```python
from build123d import *

# Parameters (mm, degrees)
SKETCH2_R          = 11.18
SKETCH2_R_2        = 7.615
CUT_EXTRUDE1_DEPTH = 18
FILLET1_R          = 0.8


with BuildPart() as part:
    # Sketch1 → Revolve1 (revolve)
    with BuildSketch(Plane(origin=(0, 0, 0), x_dir=(0, 0, -1), z_dir=(1, 0, 0)), mode=Mode.PRIVATE) as revolve1_sk:
        with BuildLine():
            Line((12.33, 64), (12.33, 44))
            Line((12.33, 44), (10, 44))
            ThreePointArc((10, 44), (8.585786438, 43.414213562), (8, 42))
            Line((8, 42), (8, 21.197712361))
            Line((8, 21.197712361), (9.005, 20))
            Line((9.005, 20), (11.005, 20))
            Line((11.005, 20), (11.005, 0))
            Line((11.005, 0), (7.73, 0))
            Line((7.73, 0), (7.73, 16))
            Line((7.73, 16), (6.5, 17.465856919))
            Line((6.5, 17.465856919), (6.5, 25.465856919))
            Line((6.5, 25.465856919), (4.5, 29.465856919))
            Line((4.5, 29.465856919), (4.5, 37.465856919))
            Line((4.5, 37.465856919), (6.5, 45.465856919))
            Line((6.5, 45.465856919), (6.5, 64))
            Line((6.5, 64), (12.33, 64))
        make_face()
    revolve(revolve1_sk.sketch.rotate(Axis((0, 34.050123762, 0), (0, -1, 0)), 180), axis=Axis((0, 34.050123762, 0), (0, -1, 0)))

    # Sketch2 → Cut-Extrude1 (cut)
    with BuildSketch(Plane(origin=(0, 64, 0), x_dir=(1, 0, 0), z_dir=(0, 1, 0))):
        with Locations(Location((0, 0, 0), (0, 0, 270))):
            Circle(SKETCH2_R)
        with Locations(Location((0, 0, 0), (0, 0, 270))):
            Circle(SKETCH2_R_2, mode=Mode.SUBTRACT)
    extrude(amount=-CUT_EXTRUDE1_DEPTH, mode=Mode.SUBTRACT)

    # Fillet1
    fillet1_edges = [part.edges().sort_by_distance(p)[0] for p in [
        (0, 64, -11.18),
        (0, 64, -7.615),
    ]]
    fillet(fillet1_edges, radius=FILLET1_R)


solid = part.part
```
Geometry check sheet. Reference: the model listing, model coordinates, mm. A direction names the side the tool comes from. Round coordinates to 2 decimals unless told otherwise and drop trailing zeros. Loops run counter-clockwise (first coordinate to the right, second up) from the corner with the lowest first, then second, coordinate; pieces in that order, holes last. Notation, with made-up numbers: (-19, 32.25) -> (29, 32.25) arc R10 ccw to (29, 44.25) -> close; hole circle Ø6 at (-40, 29). An arc over 180 degrees is marked (long way). Use a Markdown table: item, result.
(1) Set-up check for faces 1 (the cylindrical face through (-3.04, 33.52, -3.32)), 2 (the flat face through (-7, 46, 5)), 3 (the cylindrical face through (4.704, 8.112, -6.134)), 4 (the flat face through (-10.104, 44, -0.971)): record each of +Z, -Z, +X, -X, +Y, -Y from which the full face is reachable in a straight line by a thin tool's end or side.
Calculated:
| item | result |
|---|---|
| face 1 | +Y, -Y |
| face 2 | +Y |
| face 3 | -Y |
| face 4 | none |
(2) Go/stop test with flat-tipped pins: P1, Ø5, axis at x = 3, y = 13.5, coming from the -Z side; P2, Ø6, axis at y = 38.5, z = 8.5, coming from the +X side; P3, Ø2, axis at x = 5, y = 27.5, coming from the -Z side; P4, Ø8, axis at x = 0, z = 0, coming from the +Y side. Record where each tip stops, or that it passes through.
Calculated:
| item | result |
|---|---|
| P1 | z = -10.99 |
| P2 | x = 5.81 |
| P3 | z = -6.93 |
| P4 | through |
(3) Scan lines: probe 1 along X at (y, z) = (52.25, 0) (3 decimals); probe 2 along Y at (x, z) = (-4.75, -9); probe 3 along X at (y, z) = (60.5, 3.75). Record each from-to range of solid material in increasing order.
Calculated:
| item | result |
|---|---|
| probe 1 | -12.33 to -11.18, -7.615 to -6.5, 6.5 to 7.615, 11.18 to 12.33 |
| probe 2 | 0 to 20, 44 to 46 |
| probe 3 | -11.75 to -10.53, -6.63 to -5.31, 5.31 to 6.63, 10.53 to 11.75 |
(4) Mould release check, pull along Y, two halves, no side actions. Record for faces 5 (the conical face through (5.166, 40.633, -1.147)), 6 (the flat face through (9, 20, -2)), 7 (the cylindrical face through (-12.225, 53.86, -1.605)): released by +Y, released by -Y, zero draft, split by the parting line, or undercut.
Calculated:
| item | result |
|---|---|
| face 5 | released by +Y |
| face 6 | undercut |
| face 7 | zero draft |
(5) Sectioned sample at C-C (y = 6.5). Enter the section's corners in (x, z) (3 decimals).
Calculated:
| item | result |
|---|---|
| outline | circle Ø22.01 at (0, 0); hole circle Ø15.46 at (0, 0) |
(6) Sectioned sample at B-B (y = 34.5). Enter the section's corners in (x, z).
Calculated:
| item | result |
|---|---|
| outline | circle Ø16 at (0, 0); hole circle Ø9 at (0, 0) |
(7) Sectioned sample at A-A (y = 48). Enter the section's corners in (x, z) (3 decimals).
Calculated:
| item | result |
|---|---|
| outline | circle Ø24.66 at (0, 0); circle Ø15.23 at (0, 0); hole circle Ø22.36 at (0, 0); hole circle Ø13 at (0, 0) |
